Design review of the part built by this model. Coordinates are the model's own, in mm. A direction names the side the tool comes from. Give positions to 0.01 mm unless a question says otherwise; leave off trailing zeros. Order: outer loops, then holes, each group sorted by start corner. A loop starts at its lowest first (then second) coordinate and runs counter-clockwise, first axis right, second up. Notation, with made-up numbers: M 8,49.5 L 24,49.5 A14 cw 24,54.5 Z; hole C 20,51 d8. An arc over 180 degrees is marked long. Answer as a JSON object with one key per item and string values.
Autodesk Inventor part; units mm, degrees
ref_plane "YZ Plane" through (0, 0, 0) normal (1, 0, 0) x (0, 1, 0)
ref_plane "XZ Plane" through (0, 0, 0) normal (0, 1, 0) x (-1, 0, 0)
ref_plane "XY Plane" through (0, 0, 0) normal (0, 0, 1) x (1, 0, 0)
sketch "Sketch1" plane through (0, 0, 0) normal (0, 1, 0) x (-1, 0, 0)
  line L0 (0, -2.6558) -> (-2.3, -1.3279)
  line L1 (-2.3, -1.3279) -> (-2.3, 1.3279)
  line L2 (-2.3, 1.3279) -> (0, 2.6558)
  line L3 (0, 2.6558) -> (2.3, 1.3279)
  line L4 (2.3, 1.3279) -> (2.3, -1.3279)
  line L5 (2.3, -1.3279) -> (0, -2.6558)
  point P0 (0, 0)
  point P1 (0, 0)
  dimension "d0" = 4.6
extrude "Extrusion1" add sketch "Sketch1" along normal blind 20
sketch "Sketch2" plane through (0, 20, 0) normal (0, 1, 0) x (1, 0, 0)
  circle A0 centre (0, 0) radius 1.5
  dimension "d3" = 3
extrude "Extrusion2" cut sketch "Sketch2" against normal blind 15
sketch "Sketch3" plane through (0, 0, 0) normal (0, -1, 0) x (1, 0, 0)
  circle A0 centre (0, 0) radius 1.5
  dimension "d6" = 3
extrude "Extrusion3" add sketch "Sketch3" along normal blind 6
properties part number "Separador-M3-20mm-Pin" material "Stainless Steel"
(1) We need section A-A (y = 14.5). Write out the cut boundary in (x, z).
Checked values:
{"outline": "M -2.3,-1.33 L 0,-2.66 L 2.3,-1.33 L 2.3,1.33 L 0,2.66 L -2.3,1.33 Z; hole C 0,0 d3"}
(2) We need section D-D (y = 4.5). Write out the cut boundary in (x, z).
Checked values:
{"outline": "M -2.3,-1.33 L 0,-2.66 L 2.3,-1.33 L 2.3,1.33 L 0,2.66 L -2.3,1.33 Z"}
(3) Insertion check: pin 1 (0.9 mm diameter, centred on x = 0, z = 0, fed in from +Y); pin 2 (2 mm diameter, centred on x = 0, y = -3, fed in from +Z). Each pin has a flat end and moves straight along its axis. Give the tip position at first contact, or say it passes through.
Checked values:
{"pin 1": "stops at y = 5", "pin 2": "stops at z = 1.5"}
(4) We need section B-B (z = 0). Write out the cut boundary in (x, y).
Checked values:
{"outline": "M -2.3,0 L -1.5,0 L -1.5,-6 L 1.5,-6 L 1.5,0 L 2.3,0 L 2.3,20 L 1.5,20 L 1.5,5 L -1.5,5 L -1.5,20 L -2.3,20 Z"}
(5) To check wall thickness, follow L1, parallel to X at y = 12.25, z = 0; L2, parallel to Y at x = 0.85, z = 0.2; L3, parallel to Y at x = -0.1, z = -2.25. State the ranges of each line that lie inside material, in increasing order. Write a range as from..to.
Checked values:
{"L1": "x = -2.3..-1.5, 1.5..2.3", "L2": "y = -6..5", "L3": "y = 0..20"}
(6) We need section C-C (x = -1). Write out the cut boundary in (y, z), plus the area to 3 significant figures.
Checked values:
{"outline": "M -6,-1.12 L 0,-1.12 L 0,-2.08 L 20,-2.08 L 20,-1.12 L 5,-1.12 L 5,1.12 L 20,1.12 L 20,2.08 L 0,2.08 L 0,1.12 L -6,1.12 Z", "area": "63.0 mm^2"}
(7) Tool access review of faces 4 (the flat face through (2, 20, 0)), 5 (the cylindrical face through (-1.5, 12.6, -0.07)), 6 (the cylindrical face through (-1.5, -2.96, -0.07)): name each direction out of +Z, -Z, +X, -X, +Y, -Y from which nothing blocks a thin tool from reaching the whole face with its end or side.
Checked values:
{"face 4": "+Z, -Z, +X, -X, +Y", "face 5": "+Y", "face 6": "-Y"}
(8) Draft analysis for pull direction Z (two halves, no side actions). For faces 1 (the flat face through (-1.17, 9.86, -1.98)), 2 (the flat face through (0, -6, 0)), 3 (the flat face through (0, 5, 0)), state which applies: +Z half, -Z half, draft (parallel to the pull), parting line (faces both ways), or undercut.
Checked values:
{"face 1": "-Z half", "face 2": "draft", "face 3": "undercut"}
